Input: part model. Units: mm. Frame: model coordinates. A direction names the side the tool comes from. Round coordinates to 2 decimals unless told otherwise and drop trailing zeros. Loops run counter-clockwise (first coordinate to the right, second up) from the corner with the lowest first, then second, coordinate; pieces in that order, holes last. Notation, with made-up numbers: (84.25, 3.5) - (119.25, 3.5) arc R16 ccw to (119.25, 19.5) - close; hole circle Ø3 at (71.5, -19.75). An arc over 180 degrees is marked (long way). One line per question, with ' | ' between items. Start each with the question number.
Item 1: Set-up query: faces 4 (the face through (-9.93, 2.18, 9.4)), 5 (the face through (8.65, 2, -5)). Return all of +Z, -Z, +X, -X, +Y, -Y with unobstructed straight access to the full face (end or side cutting, diameter ignored); none if empty.
Item 2: Section B-B, the plane x = 0. Return loops of the section in (y, z).
Item 3: Draft query along Z for faces 1 (the face through (-10.5, 2, 0)), 2 (the face through (0, 2, -7)), 3 (the face through (0, 2, -10)). Return one class per face: pulls with the +Z half, pulls with the -Z half, needs draft (parallel to the pull), parting line crosses it, or undercut.
Item 4: Section A-A, the plane y = 1.4. Return loops of the section in (x, z), plus the area to 3 significant figures.
Item 5: Section C-C, the plane z = -6.5. Return loops of the section in (x, y).
Item 6: Section D-D, the plane z = -1. Return loops of the section in (x, y).
Item 7: Material intervals for line 1 along Z through (x, y) = (0.25, 1.6); line 2 along X through (y, z) = (1.45, -6.25); line 3 along Z through (x, y) = (-2.75, 1.6), sorted ascending.
```python
from build123d import *

# Parameters (mm, degrees)
ESBO_O2_W                = 21
ESBO_O2_H                = 20
ESBO_O2_W_2              = 17.3
ESBO_O2_H_2              = 3.3
RESSALTO_EXTRUS_O1_DEPTH = 4.3
FILETE1_R                = 1
FILETE2_R                = 1
FILETE3_R                = 2
FILETE4_R                = 2
CORTE_EXTRUS_O3_DEPTH    = 4.3


with BuildPart() as part:
    # Esboço2 → Ressalto-extrusão1 (new body)
    with BuildSketch(Plane(origin=(0, 0, 0), x_dir=(1, 0, 0), z_dir=(0, 1, 0))):
        Rectangle(ESBO_O2_W, ESBO_O2_H)
        with Locations((0, 5.35)):
            Rectangle(ESBO_O2_W_2, ESBO_O2_H_2, mode=Mode.SUBTRACT)
    extrude(amount=RESSALTO_EXTRUS_O1_DEPTH)

    # Filete1
    filete1_edges = [part.edges().sort_by_distance(p)[0] for p in [
        (10.5, 2.15, -10),
    ]]
    fillet(filete1_edges, radius=FILETE1_R)

    # Filete2
    filete2_edges = [part.edges().sort_by_distance(p)[0] for p in [
        (-10.5, 2.15, -10),
    ]]
    fillet(filete2_edges, radius=FILETE2_R)

    # Filete3
    filete3_edges = [part.edges().sort_by_distance(p)[0] for p in [
        (-10.5, 2.15, 10),
    ]]
    fillet(filete3_edges, radius=FILETE3_R)

    # Filete4
    filete4_edges = [part.edges().sort_by_distance(p)[0] for p in [
        (10.5, 2.15, 10),
    ]]
    fillet(filete4_edges, radius=FILETE4_R)

    # Esboço6 → Corte-extrusão3 (cut)
    with BuildSketch(Plane(origin=(0, 4.3, 0), x_dir=(1, 0, 0), z_dir=(0, 1, 0))):
        with BuildLine():
            ThreePointArc((-8, 0.016269222), (0, -7.983730778), (8, 0.016269222))
            ThreePointArc((8, 0.016269222), (6.516269222, 1.5), (5.032538443, 0.016269222))
            ThreePointArc((5.032538443, 0.016269222), (0, -5.016269222), (-5.032538443, 0.016269222))
            ThreePointArc((-5.032538443, 0.016269222), (-6.516269222, 1.5), (-8, 0.016269222))
        make_face()
    extrude(amount=-CORTE_EXTRUS_O3_DEPTH, mode=Mode.SUBTRACT)


solid = part.part
```
Return value:
1) face 4: +Z, -X, +Y, -Y | face 5: +Y, -Y
2) outline: (0, -10) - (4.3, -10) - (4.3, -7) - (0, -7) - close; (0, -3.7) - (4.3, -3.7) - (4.3, 5.02) - (0, 5.02) - close; (0, 7.98) - (4.3, 7.98) - (4.3, 10) - (0, 10) - close
3) face 1: needs draft | face 2: undercut | face 3: pulls with the -Z half
4) outline: (-10.5, -9) arc R1 ccw to (-9.5, -10) - (9.5, -10) arc R1 ccw to (10.5, -9) - (10.5, 8) arc R2 ccw to (8.5, 10) - (-8.5, 10) arc R2 ccw to (-10.5, 8) - close; hole (-8.65, -7) - (8.65, -7) - (8.65, -3.7) - (-8.65, -3.7) - close; hole (-8, -0.02) arc R1.48 ccw to (-5.03, -0.02) arc R5.03 cw to (5.03, -0.02) arc R1.48 ccw to (8, -0.02) arc R8 ccw to start | area: 293 mm2
5) outline: (-10.5, 0) - (-8.65, 0) - (-8.65, 4.3) - (-10.5, 4.3) - close; (8.65, 0) - (10.5, 0) - (10.5, 4.3) - (8.65, 4.3) - close
6) outline: (-10.5, 0) - (-7.63, 0) - (-7.63, 4.3) - (-10.5, 4.3) - close; (-5.41, 0) - (5.41, 0) - (5.41, 4.3) - (-5.41, 4.3) - close; (7.63, 0) - (10.5, 0) - (10.5, 4.3) - (7.63, 4.3) - close
7) line 1: -10 to -7, -3.7 to 5.01, 7.98 to 10 | line 2: -10.5 to -8.65, 8.65 to 10.5 | line 3: -10 to -7, -3.7 to 4.2, 7.5 to 10
